For this review, take the finished solid that the model builds, in its own axes (mm). A direction names the side the tool comes from. Round coordinates to 2 decimals unless told otherwise and drop trailing zeros. Write each loop counter-clockwise with the first axis right and the second up, starting at its lowest first coordinate (ties: lowest second). Pieces come first, ordered by that corner, then holes. Notation, with made-up numbers: (27.5, -14.5) -> (70.5, -14.5) arc R20 ccw to (70.5, -7.5) -> close; hole circle Ø6 at (53.5, -16). An arc over 180 degrees is marked (long way). Write each question's results on one line, items separated by ' | '. Start each with the question number.
Item 1: Add section A-A (y = 5). State the section outline as (x, z) points.
Item 2: Tool access review of faces 5 (the flat face through (4, 1, 70)), 6 (the cylindrical face through (5.765, 0.074, 44.65)), 7 (the flat face through (1, 25, 3.26)): name each direction out of +Z, -Z, +X, -X, +Y, -Y from which nothing blocks a thin tool from reaching the whole face with its end or side.
Item 3: The part is to be moulded in two halves that separate along X. For faces 1 (the cylindrical face through (4.195, 23.763, -2.958)), 2 (the flat face through (4, -2, 10)), 3 (the flat face through (4, 26, 2.25)), 4 (the flat face through (4, 47, 11)), say which applies: +X half, -X half, draft (parallel to the pull), parting line (faces both ways), or undercut.
Item 4: Clearance check with flat-ended pins moving along their axes: pin 1 (2.5 mm diameter, centred on x = 4, y = 46, fed in from +Z); pin 2 (2 mm diameter, centred on x = 1.5, z = 47, fed in from -Y); pin 3 (0.8 mm diameter, centred on x = 1, y = 33, fed in from +Z). State where each tip first meets the part, or that it passes through.
Item 5: Add section C-C (x = 4). State the section outline as (y, z) points, plus the area to 3 significant figures.
Item 6: Add section D-D (y = 25.25). State the section outline as (x, z) points, plus the area to 3 significant figures.
Item 7: To check wall thickness, follow line 1 along Y through (x, z) = (3, 17); line 2 along Z through (x, y) = (0.5, 41); line 3 along Z through (x, y) = (2.25, 39). State the ranges of each line that lie inside material, in increasing order.
Item 8: Add section B-B (z = 41). State the section outline as (x, y) points, plus the area to 3 significant figures.
Autodesk Inventor part; units mm, degrees
ref_plane "YZ Plane" through (0, 0, 0) normal (1, 0, 0) x (0, 1, 0)
ref_plane "XZ Plane" through (0, 0, 0) normal (0, 1, 0) x (-1, 0, 0)
ref_plane "XY Plane" through (0, 0, 0) normal (0, 0, 1) x (1, 0, 0)
sketch "Sketch1" plane through (0, 0, 0) normal (0, 0, 1) x (1, 0, 0)
  line L0 (0, 0) -> (8, 0)
  line L1 (8, 0) -> (8, 50.5)
  line L2 (8, 50.5) -> (0, 50.5)
  line L3 (0, 50.5) -> (0, 0)
  dimension "d0" = 8
  dimension "d1" = 50.5
extrude "Extrusion1" add sketch "Sketch1" along normal blind 20
sketch "Sketch2" plane through (0, 0, 20) normal (0, 0, 1) x (1, 0, 0)
  line L0 (8, 0) -> (8, 50.5)
  line L1 (0, 42) -> (8, 42)
  line L2 (8, 42) -> (8, 8.5)
  line L3 (8, 8.5) -> (0, 8.5)
  line L4 (0, 8.5) -> (0, 42)
  line L5 (8, 50.5) -> (0, 50.5)
  line L6 (0, 0) -> (8, 0)
  dimension "d4" = 33.5
  dimension "d5" = 8.5
  dimension "d6" = 8.5
extrude "Extrusion2" cut sketch "Sketch2" against normal blind 16.74
sketch "Sketch3" plane through (0, 0, 20) normal (0, 0, 1) x (1, 0, 0)
  line L0 (1.5, 47) -> (6.5, 47)
  line L1 (6.5, 47) -> (6.5, 3.5)
  line L2 (6.5, 3.5) -> (1.5, 3.5)
  line L3 (1.5, 3.5) -> (1.5, 47)
  line L4 (0, 50.5) -> (0, 42)
  line L5 (0, 42) -> (8, 42)
  line L6 (8, 8.5) -> (0, 8.5)
  point P0 (0, 0)
  dimension "d9" = 5
  dimension "d10" = 1.5
  dimension "d11" = 5
  dimension "d12" = 5
extrude "Extrusion3" cut sketch "Sketch3" against normal blind 17.75
sketch "Sketch4" plane through (0, 0, 20) normal (0, 0, 1) x (1, 0, 0)
  line L0 (8, 50.5) -> (0, 50.5)
  line L1 (0, 50.5) -> (8, 50.5)
  line L2 (8, 50.5) -> (8, 52.5)
  line L3 (8, 52.5) -> (0, 52.5)
  line L4 (0, 52.5) -> (0, 50.5)
  line L5 (0, 0) -> (8, 0)
  line L6 (0, 0) -> (8, 0)
  line L7 (8, 0) -> (8, -2)
  line L8 (8, -2) -> (0, -2)
  line L9 (0, -2) -> (0, 0)
  dimension "d15" = 2
extrude "Extrusion4" add sketch "Sketch4" against normal up to surface (20 mm away)
sketch "Sketch5" plane through (0, 0, 20) normal (0, 0, 1) x (1, 0, 0)
  circle A0 centre (4.1899, 49.75) radius 2.25
  circle A1 centre (3.6194, 0.75) radius 2.25
  line L0 (0, -2) -> (8, -2)
  line L1 (6.5, 3.5) -> (1.5, 3.5)
  line L2 (1.5, 47) -> (6.5, 47)
  point P0 (0, 0)
  dimension "d18" = 5.5
  dimension "d19" = 4.5
  dimension "d20" = 2.75
  dimension "d21" = 2.75
extrude "Extrusion5" add sketch "Sketch5" along normal blind 50
sketch "Sketch6" plane through (0, 0, 0) normal (0, 0, -1) x (-1, 0, 0)
  line L0 (0, -2) -> (0, 52.5)
  line L1 (-8, -2) -> (-8, 52.5)
  circle A0 centre (-4, 25.25) radius 1.5
  line L2 (-8, -2) -> (0, -2)
  line L3 (0, 52.5) -> (-8, 52.5)
  point P0 (0, 0)
  dimension "d24" = 8
  dimension "d25" = 4
  dimension "d26" = 3
  dimension "d27" = 54.5
  dimension "d28" = 27.25
extrude "Extrusion6" add sketch "Sketch6" along normal blind 6 contours A0
properties part number "Stand Lower covet"
Responses:
1) outline: (0, 0) -> (8, 0) -> (8, 20) -> (6.5, 20) -> (6.5, 2.25) -> (1.5, 2.25) -> (1.5, 20) -> (0, 20) -> close
2) face 5: +Z, +X, -X, +Y, -Y | face 6: +Z | face 7: +Z, +X, -X
3) face 1: parting line | face 2: draft | face 3: undercut | face 4: undercut
4) pin 1: stops at z = 20 | pin 2: stops at y = -1.2 | pin 3: stops at z = 3.26
5) outline: (-2, 0) -> (23.75, 0) -> (23.75, -6) -> (26.75, -6) -> (26.75, 0) -> (52.5, 0) -> (52.5, 20) -> (51.99, 20) -> (51.99, 70) -> (47.51, 70) -> (47.51, 20) -> (47, 20) -> (47, 2.25) -> (3.5, 2.25) -> (3.5, 20) -> (2.97, 20) -> (2.97, 70) -> (-1.47, 70) -> (-1.47, 20) -> (-2, 20) -> close | area: 782 mm^2
6) outline: (0, 0) -> (2.5, 0) -> (2.5, -6) -> (5.5, -6) -> (5.5, 0) -> (8, 0) -> (8, 3.26) -> (6.5, 3.26) -> (6.5, 2.25) -> (1.5, 2.25) -> (1.5, 3.26) -> (0, 3.26) -> close | area: 39.0 mm^2
7) line 1: y = -2 to 3.5, 47 to 52.5 | line 2: z = 0 to 3.26 | line 3: z = 0 to 2.25
8) outline: circle Ø4.5 at (3.62, 0.75); circle Ø4.5 at (4.19, 49.75) | area: 31.8 mm^2
